from build123d import *

# Parameters (mm, degrees)
SKETCH_1_R                = 40
EXTRUDE_1_DEPTH           = 35
HOLE_WIZARD_1_D           = 6.6
HOLE_WIZARD_1_DEPTH       = 50
HOLE_WIZARD_1_CBORE_D     = 11
HOLE_WIZARD_1_CBORE_DEPTH = 6.8
HOLE_WIZARD_1_TIP         = 1.982840043
HOLE_WIZARD_M5_1_D        = 4.2
HOLE_WIZARD_M5_1_DEPTH    = 12.4
HOLE_WIZARD_M5_1_TIP      = 1.2618073
HOLE_WIZARD_M4_1_D        = 3.3
HOLE_WIZARD_M4_1_DEPTH    = 10.1
HOLE_WIZARD_M4_1_TIP      = 0.991420021
HOLE_WIZARD_M8_1_D        = 6.8
HOLE_WIZARD_M8_1_DEPTH    = 19.75
HOLE_WIZARD_M8_1_TIP      = 2.042926105
SKETCH_7_R                = 2.065
CUT_EXTRUDE_1_DEPTH       = 40


with BuildPart() as part:
    # 草图1 → 凸台-拉伸1 (new body)
    with BuildSketch(Plane(origin=(0, 0, 0), x_dir=(1, 0, 0), z_dir=(0, 1, 0))):
        Circle(SKETCH_1_R)
    extrude(amount=EXTRUDE_1_DEPTH)

    # 打孔尺寸(%根据)内六角圆柱头螺钉的类型1
    with Locations(Plane(origin=(-20, 35, -20), x_dir=(0, 0, 1), z_dir=(0, 1, 0))):
        with Locations((0, 0), (0, 40), (40, 40), (40, 0)):
            CounterBoreHole(HOLE_WIZARD_1_D / 2, HOLE_WIZARD_1_CBORE_D / 2, HOLE_WIZARD_1_CBORE_DEPTH, depth=HOLE_WIZARD_1_DEPTH)
            with Locations((0, 0, -(HOLE_WIZARD_1_DEPTH + HOLE_WIZARD_1_TIP / 2))):  # 118° drill point
                Cone(0, HOLE_WIZARD_1_D / 2, HOLE_WIZARD_1_TIP, mode=Mode.SUBTRACT)

    # M5 螺纹孔1
    with Locations(Plane(origin=(0, 35, -12.5), x_dir=(0, 0, 1), z_dir=(0, 1, 0))):
        with Locations((0, 0), (25, 0), (12.5, 12.5), (12.5, -12.5)):
            Hole(HOLE_WIZARD_M5_1_D / 2, depth=HOLE_WIZARD_M5_1_DEPTH)
            with Locations((0, 0, -(HOLE_WIZARD_M5_1_DEPTH + HOLE_WIZARD_M5_1_TIP / 2))):  # 118° drill point
                Cone(0, HOLE_WIZARD_M5_1_D / 2, HOLE_WIZARD_M5_1_TIP, mode=Mode.SUBTRACT)

    # M4 螺纹孔1
    with Locations(Plane(origin=(-8.838834765, 35, -8.838834765), x_dir=(0, 0, 1), z_dir=(0, 1, 0))):
        with Locations((0, 0), (0.495114697, 17.182554833), (17.67766953, 17.67766953), (17.67766953, 0)):
            Hole(HOLE_WIZARD_M4_1_D / 2, depth=HOLE_WIZARD_M4_1_DEPTH)
            with Locations((0, 0, -(HOLE_WIZARD_M4_1_DEPTH + HOLE_WIZARD_M4_1_TIP / 2))):  # 118° drill point
                Cone(0, HOLE_WIZARD_M4_1_D / 2, HOLE_WIZARD_M4_1_TIP, mode=Mode.SUBTRACT)

    # M8 螺纹孔1
    with Locations(Plane.ZX.offset(35)):
        with Locations((0, 0)):
            Hole(HOLE_WIZARD_M8_1_D / 2, depth=HOLE_WIZARD_M8_1_DEPTH)
            with Locations((0, 0, -(HOLE_WIZARD_M8_1_DEPTH + HOLE_WIZARD_M8_1_TIP / 2))):  # 118° drill point
                Cone(0, HOLE_WIZARD_M8_1_D / 2, HOLE_WIZARD_M8_1_TIP, mode=Mode.SUBTRACT)

    # 草图7 → 切除-拉伸1 (cut)
    with BuildSketch(Plane(origin=(-15.307337295, 35, -36.9551813), x_dir=(-0.923879533, 0, 0.382683432), z_dir=(-0.382683432, 0, -0.923879533))):
        with Locations((0, -10)):
            Circle(SKETCH_7_R)
    extrude(amount=-CUT_EXTRUDE_1_DEPTH, mode=Mode.SUBTRACT)


solid = part.part
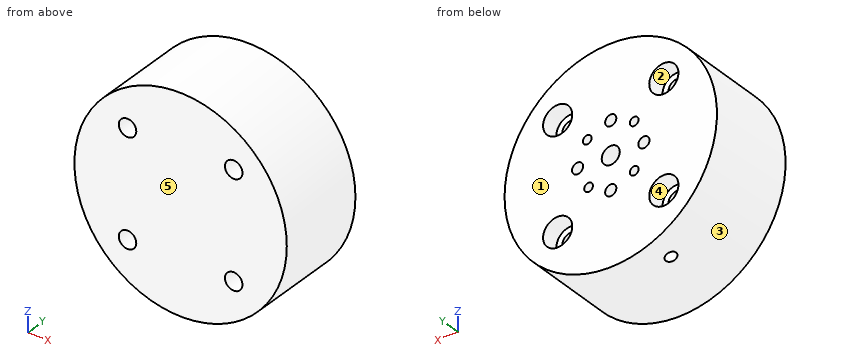
Source: CAD feature listing. Evaluate the final solid. Frame: model axes, mm. Face numbers are marked on the shaded views. A direction names the side the tool comes from. Give positions to 0.01 mm unless a question says otherwise; leave off trailing zeros. Write each loop counter-clockwise with the first axis right and the second up, starting at its lowest first coordinate (ties: lowest second). Pieces come first, ordered by that corner, then holes. Notation, with made-up numbers: M 79.25,8.25 L 104.25,8.25 A16 cw 104.25,29.25 Z; hole C 66,77 d9. An arc over 180 degrees is marked long. Return JSON: item names as keys, results as strings. Group by question number.
1) Cut plane B-B, the plane x = 20. Output: boundary loops of the cut face in (y, z), then the cut area to 3 significant figures.
2) Cut plane C-C, the plane y = 11. Output: boundary loops of the cut face in (x, z), then the cut area to 3 significant figures.
3) Draft query along X for the marked faces 3, 4 and 5. Return one class per face: released by +X, released by -X, zero draft, split by the parting line, or undercut.
4) Set-up query: the marked faces 1 and 2. Return all of +Z, -Z, +X, -X, +Y, -Y with unobstructed straight access to the full face (end or side cutting, diameter ignored); none if empty.
5) Cut plane A-A, the plane y = 18. Output: boundary loops of the cut face in (x, z).
6) First-contact query: pin 1 Ø10 at (x, y) = (23, 24) entering from -Z; pin 2 Ø11 at (x, z) = (0, 0) entering from +Y; pin 3 Ø3 at (x, z) = (-8.84, -8.84) entering from +Y; pin 4 Ø5.5 at (x, z) = (-22, -20.5) entering from +Y. Flat tips, straight axial feed; report the tip coordinate or a pass-through.
7) Cut plane D-D, the plane z = 21.5. Output: boundary loops of the cut face in (x, y), then the cut area to 3 significant figures.
8) Ray query, L1, parallel to X at y = 27.75, z = 0; L2, parallel to Z at x = -1, y = 32. Return the intervals inside material, ascending.
Data:
{
 "1": {"outline": "M 0,-34.64 L 35,-34.64 L 35,-25.5 L 28.2,-25.5 L 28.2,-23.3 L 0,-23.3 Z; M 0,-16.7 L 28.2,-16.7 L 28.2,-14.5 L 35,-14.5 L 35,14.5 L 28.2,14.5 L 28.2,16.7 L 0,16.7 Z; M 0,23.3 L 28.2,23.3 L 28.2,25.5 L 35,25.5 L 35,34.64 L 0,34.64 Z", "area": "1,900 mm²"},
 "2": {"outline": "C 0,0 d80; hole C -20,-20 d6.6; hole C -20,20 d6.6; hole C 20,-20 d6.6; hole C 20,20 d6.6", "area": "4,890 mm²"},
 "3": {"face 3": "split by the parting line", "face 4": "undercut", "face 5": "zero draft"},
 "4": {"face 1": "+Z, -Z, +X, -X, +Y", "face 2": "+Y"},
 "5": {"outline": "C 0,0 d80; hole C -20,-20 d6.6; hole C -20,20 d6.6; hole C 0,0 d6.8; hole C 20,-20 d6.6; hole C 20,20 d6.6"},
 "6": {"pin 1": "stops at z = -35.72", "pin 2": "stops at y = 35", "pin 3": "stops at y = 24.81", "pin 4": "stops at y = 28.2"},
 "7": {"outline": "M -33.73,0 L -22.94,0 L -22.94,28.2 L -25.29,28.2 L -25.29,35 L -33.73,35 Z; M -17.06,0 L 17.06,0 L 17.06,28.2 L 14.71,28.2 L 14.71,35 L -14.71,35 L -14.71,28.2 L -17.06,28.2 Z; M 22.94,0 L 33.73,0 L 33.73,35 L 25.29,35 L 25.29,28.2 L 22.94,28.2 Z", "area": "1,890 mm²"},
 "8": {"L1": "x = -40 to -14.6, -10.4 to -3.4, 3.4 to 10.4, 14.6 to 40", "L2": "z = -39.99 to -14.35, -10.65 to -3.25, 3.25 to 10.65, 14.35 to 39.99"}
}
